For this review, take the finished solid that the model builds, in its own axes (mm). Give positions to 0.01 mm unless a question says otherwise; leave off trailing zeros. Write each loop counter-clockwise with the first axis right and the second up, starting at its lowest first coordinate (ties: lowest second). Pieces come first, ordered by that corner, then holes.
1) Draft analysis for pull direction X (two halves, no side actions). For faces 1 (the face through (-23.668, 1.565, -33.446)), 2 (the face through (34, 0, -18)), 3 (the face through (72.508, 1.565, -34.946)), 4 (the face through (-25.771, 1.565, -2.542)), state which applies: pulls with the +X half, pulls with the -X half, needs draft (parallel to the pull), parting line crosses it, or undercut.
2) We need section C-C on x = 75.5. Give the boundary of the cut face in (y, z) (3 decimals).
3) We need section B-B on y = 2.1. Give the number of separate pieces and of enclosed holes in the cut face, and give its area (3 significant figures).
4) Wall thickness on line 1 along X through (y, z) = (0.8, -13); line 2 along X through (y, z) = (2.9, -8.5); line 3 along Z through (x, y) = (21.5, 1.75): over which ranges is each line inside the solid? List them lowest first.
5) For P1, Ø1, axis at y = 2.5, z = -8.5, coming from the -X side; P2, Ø1, axis at x = 37, y = 2.5, coming from the +Z side, all flat-tipped, find the tip position at first contact; note any pin that passes through.
6) We need section D-D on x = 13. Give the boundary of the cut face in (y, z) (3 decimals).
7) We need section A-A on x = -18. Give the boundary of the cut face in (y, z) (3 decimals), and give its area (3 significant figures).
Autodesk Inventor part; units mm, degrees
ref_plane "YZ Plane" through (0, 0, 0) normal (1, 0, 0) x (0, 1, 0)
ref_plane "XZ Plane" through (0, 0, 0) normal (0, 1, 0) x (-1, 0, 0)
ref_plane "XY Plane" through (0, 0, 0) normal (0, 0, 1) x (1, 0, 0)
sketch "Sketch1" plane through (0, 0, 0) normal (0, 1, 0) x (-1, 0, 0)
  line L0 (-28.6419, -11.7592) -> (-388.4279, -11.7592) construction
  arc A0 (-111.6419, 3.957) -> (-111.6419, -27.4755) centre (-108.6419, -11.7592) ccw
  arc A1 (37.9831, -35.6153) -> (37.9831, 12.0968) centre (35.3581, -11.7592) ccw
  line L1 (-25.2513, -42.5733) -> (37.9831, -35.6153)
  line L2 (-25.2513, 19.0548) -> (37.9831, 12.0968)
  line L3 (-34.4544, -42.2094) -> (-111.6419, -27.4755)
  line L4 (-111.6419, 3.957) -> (-34.4544, 18.691)
  arc A2 (-25.2513, 19.0548) -> (-34.4544, 18.691) centre (-28.6419, -11.7592) ccw
  arc A3 (-34.4544, -42.2094) -> (-25.2513, -42.5733) centre (-28.6419, -11.7592) ccw
  circle A4 centre (-108.6419, -11.7592) radius 7
  circle A5 centre (35.3581, -11.7592) radius 7
  circle A6 centre (-28.6419, -11.7592) radius 7
  circle A7 centre (27.3581, -3.7592) radius 2
  circle A8 centre (27.3581, -19.7592) radius 2
  circle A9 centre (43.3581, -19.7592) radius 2
  circle A10 centre (43.3581, -3.7592) radius 2
  circle A11 centre (35.3581, -11.7592) radius 11.3137 construction
  circle A12 centre (-108.6419, -11.7592) radius 43 construction
  circle A13 centre (-28.6419, -11.7592) radius 55 construction
  circle A14 centre (22.5928, -31.7592) radius 2
  circle A15 centre (22.5928, 8.2408) radius 2
  circle A16 centre (-36.6419, -19.7592) radius 2
  circle A17 centre (-20.6419, -19.7592) radius 2
  circle A18 centre (-20.6419, -3.7592) radius 2
  circle A19 centre (-36.6419, -3.7592) radius 2
  circle A20 centre (11.3581, -19.7592) radius 2
  circle A21 centre (11.3581, -3.7592) radius 2
  circle A22 centre (19.3581, -11.7592) radius 3.6
  dimension "d21" = 110
  dimension "d3" = 32
  dimension "d4" = 80
  dimension "d5" = 48
  dimension "d6" = 64
  dimension "d7" = 14
  dimension "d8" = 14
  dimension "d9" = 14
  dimension "d12" = 4
  dimension "d15" = 360
  dimension "d19" = 86
  dimension "d22" = 4
  dimension "d23" = 20
  dimension "d24" = 8
  dimension "d25" = 8
  dimension "d26" = 4
  dimension "d29" = 360
  dimension "d31" = 8
  dimension "d32" = 4
  dimension "d33" = 16
  dimension "d34" = 7.2
  dimension "d35" = 8
extrude "Extrusion1" add sketch "Sketch1" along normal blind 3.175
properties part number "bean" material "Aluminum 6061"
Results list:
1. face 1: undercut
1. face 2: needs draft
1. face 3: pulls with the +X half
1. face 4: undercut
2. outline: (0, -34.374) - (3.175, -34.374) - (3.175, 10.856) - (0, 10.856) - close
3. separate pieces: 1
3. enclosed holes: 16
3. area: 8,020 mm2
4. line 1: x = -59.33 to -42.25, -28.47 to -22.74, -15.98 to 21.75, 35.53 to 101.75, 115.53 to 124.59
4. line 2: x = -59.14 to -41.55, -29.16 to -20.89, -17.83 to 22.45, 34.84 to 102.45, 114.84 to 124.31
4. line 3: z = -42.16 to -21.57, -17.95 to -5.57, -1.95 to 18.64
5. P1: stops at x = -59.2
5. P2: stops at z = 18.3
6. outline: (0, -41.225) - (3.175, -41.225) - (3.175, 17.707) - (0, 17.707) - close
7. outline: (0, -37.814) - (3.175, -37.814) - (3.175, -15.093) - (0, -15.093) - close; (0, -8.425) - (3.175, -8.425) - (3.175, 14.296) - (0, 14.296) - close
7. area: 144 mm2
